Source: CAD feature listing. Evaluate the final solid. Frame: model axes, mm. A direction names the side the tool comes from. Round coordinates to 2 decimals unless told otherwise and drop trailing zeros. Loops run counter-clockwise (first coordinate to the right, second up) from the corner with the lowest first, then second, coordinate; pieces in that order, holes last. Notation, with made-up numbers: (34.25, 22) - (53.25, 22) arc R30 cw to (53.25, 45) - close; hole circle Ø8 at (12, 25). An arc over 180 degrees is marked (long way). Use CSV: the item, a comma, the result in double quotes. Start each with the question number.
from build123d import *

# Parameters (mm, degrees)
F1_DEPTH = 3.048
F3_DEPTH = 3.048
F5_DEPTH = 3.048


with BuildPart() as f1:
    # F0 (on Front) → F1 (new body)
    with BuildSketch(Plane.XZ):
        with BuildLine():
            Line((-27.215604, 61.783131), (-27.215604, -68.822387))
            ThreePointArc((-27.215604, -68.822387), (-26.099681, -71.516464), (-23.405604, -72.632387))
            Line((-23.405604, -72.632387), (-2.464669, -72.632387))
            Line((-2.464669, -72.632387), (-2.464669, -64.140432))
            Line((-2.464669, -64.140432), (-24.693408, -64.140432))
            ThreePointArc((-24.693408, -64.140432), (-25.232223, -63.917247), (-25.455408, -63.378432))
            Line((-25.455408, -63.378432), (-25.455408, -25.846069))
            ThreePointArc((-25.455408, -25.846069), (-25.232223, -25.307254), (-24.693408, -25.084069))
            Line((-24.693408, -25.084069), (-2.464669, -25.084069))
            Line((-2.464669, -25.084069), (-2.464669, -19.391987))
            Line((-2.464669, -19.391987), (-5.690682, -19.391987))
            ThreePointArc((-5.690682, -19.391987), (-6.229498, -19.168803), (-6.452682, -18.629987))
            Line((-6.452682, -18.629987), (-6.452682, 29.59835))
            ThreePointArc((-6.452682, 29.59835), (-6.229498, 30.137166), (-5.690682, 30.36035))
            Line((-5.690682, 30.36035), (-2.287077, 30.36035))
            Line((-2.287077, 30.36035), (-2.287077, 65.593131))
            Line((-2.287077, 65.593131), (-23.405604, 65.593131))
            ThreePointArc((-23.405604, 65.593131), (-26.099681, 64.477208), (-27.215604, 61.783131))
        make_face()
        with BuildLine():
            ThreePointArc((-25.455408, 8.798287), (-25.232223, 9.337102), (-24.693408, 9.560287))
            Line((-24.693408, 9.560287), (-17.513451, 9.560287))
            ThreePointArc((-17.513451, 9.560287), (-16.974636, 9.337102), (-16.751451, 8.798287))
            Line((-16.751451, 8.798287), (-16.751451, -1.699802))
            ThreePointArc((-16.751451, -1.699802), (-16.974636, -2.238618), (-17.513451, -2.461802))
            Line((-17.513451, -2.461802), (-24.693408, -2.461802))
            ThreePointArc((-24.693408, -2.461802), (-25.232223, -2.238618), (-25.455408, -1.699802))
            Line((-25.455408, -1.699802), (-25.455408, 8.798287))
        make_face(mode=Mode.SUBTRACT)
        with BuildLine():
            ThreePointArc((-25.455408, -7.460729), (-25.232223, -6.921914), (-24.693408, -6.698729))
            Line((-24.693408, -6.698729), (-16.028815, -6.698729))
            ThreePointArc((-16.028815, -6.698729), (-15.49, -6.475544), (-15.266815, -5.936729))
            Line((-15.266815, -5.936729), (-15.266815, 26.060438))
            ThreePointArc((-15.266815, 26.060438), (-15.043631, 26.599254), (-14.504815, 26.822438))
            Line((-14.504815, 26.822438), (-10.855766, 26.822438))
            ThreePointArc((-10.855766, 26.822438), (-10.316951, 26.599254), (-10.093766, 26.060438))
            Line((-10.093766, 26.060438), (-10.093766, -18.629987))
            ThreePointArc((-10.093766, -18.629987), (-10.316951, -19.168803), (-10.855766, -19.391987))
            Line((-10.855766, -19.391987), (-24.693408, -19.391987))
            ThreePointArc((-24.693408, -19.391987), (-25.232223, -19.168803), (-25.455408, -18.629987))
            Line((-25.455408, -18.629987), (-25.455408, -7.460729))
        make_face(mode=Mode.SUBTRACT)
        with BuildLine():
            ThreePointArc((-25.455408, 26.060438), (-25.232223, 26.599254), (-24.693408, 26.822438))
            Line((-24.693408, 26.822438), (-17.451537, 26.822438))
            ThreePointArc((-17.451537, 26.822438), (-16.912722, 26.599254), (-16.689537, 26.060438))
            Line((-16.689537, 26.060438), (-16.689537, 15.614866))
            ThreePointArc((-16.689537, 15.614866), (-16.912722, 15.07605), (-17.451537, 14.852866))
            Line((-17.451537, 14.852866), (-24.693408, 14.852866))
            ThreePointArc((-24.693408, 14.852866), (-25.232223, 15.07605), (-25.455408, 15.614866))
            Line((-25.455408, 15.614866), (-25.455408, 26.060438))
        make_face(mode=Mode.SUBTRACT)
        with BuildLine():
            Line((-25.455408, 31.034609), (-25.455408, 56.824335))
            ThreePointArc((-25.455408, 56.824335), (-25.232223, 57.36315), (-24.693408, 57.586335))
            Line((-24.693408, 57.586335), (-6.186478, 57.586335))
            ThreePointArc((-6.186478, 57.586335), (-5.647663, 57.36315), (-5.424478, 56.824335))
            Line((-5.424478, 56.824335), (-5.424478, 37.310197))
            ThreePointArc((-5.424478, 37.310197), (-5.647663, 36.771382), (-6.186478, 36.548197))
            Line((-6.186478, 36.548197), (-10.055168, 36.548197))
            ThreePointArc((-10.055168, 36.548197), (-10.593984, 36.325013), (-10.817168, 35.786197))
            Line((-10.817168, 35.786197), (-10.817168, 31.034609))
            ThreePointArc((-10.817168, 31.034609), (-11.040353, 30.495793), (-11.579168, 30.272609))
            Line((-11.579168, 30.272609), (-24.693408, 30.272609))
            ThreePointArc((-24.693408, 30.272609), (-25.232223, 30.495793), (-25.455408, 31.034609))
        make_face(mode=Mode.SUBTRACT)
        with BuildLine():
            Line((-1.799683, -19.391987), (-1.799683, -72.632387))
            Line((-1.799683, -72.632387), (22.221839, -72.632387))
            ThreePointArc((22.221839, -72.632387), (24.915916, -71.516464), (26.031839, -68.822387))
            Line((26.031839, -68.822387), (26.031839, 61.783131))
            ThreePointArc((26.031839, 61.783131), (24.915916, 64.477208), (22.221839, 65.593131))
            Line((22.221839, 65.593131), (-1.654555, 65.593131))
            Line((-1.654555, 65.593131), (-1.654555, 57.586335))
            Line((-1.654555, 57.586335), (22.565058, 57.586335))
            ThreePointArc((22.565058, 57.586335), (23.103874, 57.36315), (23.327058, 56.824335))
            Line((23.327058, 56.824335), (23.327058, 37.38084))
            ThreePointArc((23.327058, 37.38084), (23.103874, 36.842025), (22.565058, 36.61884))
            Line((22.565058, 36.61884), (-1.516778, 36.61884))
            Line((-1.516778, 36.61884), (-1.516778, 30.44359))
            Line((-1.516778, 30.44359), (4.297159, 30.44359))
            ThreePointArc((4.297159, 30.44359), (4.835975, 30.220406), (5.059159, 29.68159))
            Line((5.059159, 29.68159), (5.059159, -18.629987))
            ThreePointArc((5.059159, -18.629987), (4.835975, -19.168803), (4.297159, -19.391987))
            Line((4.297159, -19.391987), (-1.799683, -19.391987))
        make_face()
        with BuildLine():
            Line((23.327058, -19.723452), (23.327058, -63.378432))
            ThreePointArc((23.327058, -63.378432), (23.103874, -63.917247), (22.565058, -64.140432))
            Line((22.565058, -64.140432), (4.102913, -64.140432))
            ThreePointArc((4.102913, -64.140432), (3.564097, -63.917247), (3.340913, -63.378432))
            Line((3.340913, -63.378432), (3.340913, -26.143166))
            ThreePointArc((3.340913, -26.143166), (3.564097, -25.604351), (4.102913, -25.381166))
            Line((4.102913, -25.381166), (8.884725, -25.381166))
            Line((8.884725, -25.381166), (8.884725, -19.723452))
            ThreePointArc((8.884725, -19.723452), (9.10791, -19.184637), (9.646725, -18.961452))
            Line((9.646725, -18.961452), (22.565058, -18.961452))
            ThreePointArc((22.565058, -18.961452), (23.103874, -19.184637), (23.327058, -19.723452))
        make_face(mode=Mode.SUBTRACT)
        with BuildLine():
            Line((16.206523, -3.277048), (22.565058, -3.277048))
            ThreePointArc((22.565058, -3.277048), (23.103874, -3.500233), (23.327058, -4.039048))
            Line((23.327058, -4.039048), (23.327058, -14.328273))
            ThreePointArc((23.327058, -14.328273), (23.103874, -14.867088), (22.565058, -15.090273))
            Line((22.565058, -15.090273), (16.206523, -15.090273))
            ThreePointArc((16.206523, -15.090273), (15.667707, -14.867088), (15.444523, -14.328273))
            Line((15.444523, -14.328273), (15.444523, -4.039048))
            ThreePointArc((15.444523, -4.039048), (15.667707, -3.500233), (16.206523, -3.277048))
        make_face(mode=Mode.SUBTRACT)
        with BuildLine():
            Line((9.334675, 30.473812), (22.565058, 30.473812))
            ThreePointArc((22.565058, 30.473812), (23.103874, 30.250627), (23.327058, 29.711812))
            Line((23.327058, 29.711812), (23.327058, 18.880225))
            ThreePointArc((23.327058, 18.880225), (23.103874, 18.34141), (22.565058, 18.118225))
            Line((22.565058, 18.118225), (14.499665, 18.118225))
            ThreePointArc((14.499665, 18.118225), (13.96085, 17.89504), (13.737665, 17.356225))
            Line((13.737665, 17.356225), (13.737665, -14.725744))
            ThreePointArc((13.737665, -14.725744), (13.514481, -15.264559), (12.975665, -15.487744))
            Line((12.975665, -15.487744), (9.334675, -15.487744))
            ThreePointArc((9.334675, -15.487744), (8.79586, -15.264559), (8.572675, -14.725744))
            Line((8.572675, -14.725744), (8.572675, 29.711812))
            ThreePointArc((8.572675, 29.711812), (8.79586, 30.250627), (9.334675, 30.473812))
        make_face(mode=Mode.SUBTRACT)
        with BuildLine():
            Line((15.88612, 14.02483), (22.565058, 14.02483))
            ThreePointArc((22.565058, 14.02483), (23.103874, 13.801646), (23.327058, 13.26283))
            Line((23.327058, 13.26283), (23.327058, 2.677905))
            ThreePointArc((23.327058, 2.677905), (23.103874, 2.139089), (22.565058, 1.915905))
            Line((22.565058, 1.915905), (15.88612, 1.915905))
            ThreePointArc((15.88612, 1.915905), (15.347304, 2.139089), (15.12412, 2.677905))
            Line((15.12412, 2.677905), (15.12412, 13.26283))
            ThreePointArc((15.12412, 13.26283), (15.347304, 13.801646), (15.88612, 14.02483))
        make_face(mode=Mode.SUBTRACT)
    extrude(amount=F1_DEPTH)

    # F2 (on Front) → F3 (join)
    with BuildSketch(Plane.XZ):
        with BuildLine():
            Line((-25.056604, -74.105591), (23.872839, -74.105591))
            ThreePointArc((23.872839, -74.105591), (26.566916, -72.989667), (27.682839, -70.295591))
            Line((27.682839, -70.295591), (27.682839, 63.256334))
            ThreePointArc((27.682839, 63.256334), (26.566916, 65.950411), (23.872839, 67.066334))
            Line((23.872839, 67.066334), (-25.056604, 67.066334))
            ThreePointArc((-25.056604, 67.066334), (-27.750681, 65.950411), (-28.866604, 63.256334))
            Line((-28.866604, 63.256334), (-28.866604, -70.295591))
            ThreePointArc((-28.866604, -70.295591), (-27.750681, -72.989667), (-25.056604, -74.105591))
        make_face()
        with BuildLine():
            Line((-16.71073, -64.140432), (-24.693408, -64.140432))
            ThreePointArc((-24.693408, -64.140432), (-25.232223, -63.917247), (-25.455408, -63.378432))
            Line((-25.455408, -63.378432), (-25.455408, -25.846069))
            ThreePointArc((-25.455408, -25.846069), (-25.232223, -25.307254), (-24.693408, -25.084069))
            Line((-24.693408, -25.084069), (-16.71073, -25.084069))
            Line((-16.71073, -25.084069), (-16.71073, -64.140432))
        make_face(mode=Mode.SUBTRACT)
        with BuildLine():
            Line((-16.71073, 57.586335), (-16.71073, 30.272609))
            Line((-16.71073, 30.272609), (-24.693408, 30.272609))
            ThreePointArc((-24.693408, 30.272609), (-25.232223, 30.495793), (-25.455408, 31.034609))
            Line((-25.455408, 31.034609), (-25.455408, 56.824335))
            ThreePointArc((-25.455408, 56.824335), (-25.232223, 57.36315), (-24.693408, 57.586335))
            Line((-24.693408, 57.586335), (-16.71073, 57.586335))
        make_face(mode=Mode.SUBTRACT)
    extrude(amount=-F3_DEPTH)

    # F4 (on face) → F5 (join)
    with BuildSketch(Plane(origin=(0, 3.048, 0), x_dir=(-1, 0, 0), z_dir=(0, 1, 0))):
        with BuildLine():
            Line((-29.664039, 64.526334), (-29.664039, -71.565591))
            ThreePointArc((-29.664039, -71.565591), (-28.176141, -75.157693), (-24.584039, -76.645591))
            Line((-24.584039, -76.645591), (25.767804, -76.645591))
            ThreePointArc((25.767804, -76.645591), (29.359906, -75.157693), (30.847804, -71.565591))
            Line((30.847804, -71.565591), (30.847804, 64.526334))
            ThreePointArc((30.847804, 64.526334), (29.359906, 68.118437), (25.767804, 69.606334))
            Line((25.767804, 69.606334), (-24.584039, 69.606334))
            ThreePointArc((-24.584039, 69.606334), (-28.176141, 68.118437), (-29.664039, 64.526334))
        make_face()
    extrude(amount=F5_DEPTH)


solid = f1.part
1. Section query A-A on z = -27.5. Return the cut outline in (x, y).
2. Mould query, pull axis Z, two halves, no side actions, for faces 4 (the cylindrical face through (24.945, -1.503, 64.447)), 5 (the flat face through (-1.8, -2, -46)), 6 (the flat face through (-21, 0, 21)). Classes: +Z half, -Z half, draft (parallel to the pull), parting line (faces both ways), or undercut.
3. Reachability of faces 1 (the flat face through (-2.465, -2, -68)), 2 (the flat face through (-27.216, -2, -3)), 3 (the flat face through (-21, -2, -2.462)) from +Z, -Z, +X, -X, +Y, -Y: full face, straight path, thin tool, end or side. Return the list, or none.
4. Section query C-C on z = 43.5. Return the cut outline in (x, y).
5. Line query: line 1 along Z through (x, y) = (-22.5, 1.5); line 2 along Z through (x, y) = (-7.5, -2); line 3 along X through (y, z) = (-1.75, -10). Output: solid intervals per line, ascending.
6. Section query D-D on x = 7. Return the cut outline in (y, z).
7. Contact query for flat-ended pins moving along their axis: P1, Ø2.5, axis at x = 2, y = -1, coming from the -Z side; P2, Ø1.5, axis at y = -1.5, z = -36.5, coming from the +X side; P3, Ø1.5, axis at y = -0.5, z = 37.5, coming from the +X side. Output: stop coordinate, or through.
Values:
1,outline,"(-30.85, 3.05) - (-28.87, 3.05) - (-28.87, 0) - (-27.22, 0) - (-27.22, -3.05) - (-25.46, -3.05) - (-25.46, 3.05) - (-16.71, 3.05) - (-16.71, 0) - (-1.8, 0) - (-1.8, -3.05) - (3.34, -3.05) - (3.34, 0) - (23.33, 0) - (23.33, -3.05) - (26.03, -3.05) - (26.03, 0) - (27.68, 0) - (27.68, 3.05) - (29.66, 3.05) - (29.66, 6.1) - (-30.85, 6.1) - close"
2,face 4,"+Z half"
2,face 5,"draft"
2,face 6,"undercut"
3,face 1,"-Z, -Y"
3,face 2,"+Z, -Z, -X, -Y"
3,face 3,"-Y"
4,outline,"(-30.85, 3.05) - (-28.87, 3.05) - (-28.87, 0) - (-27.22, 0) - (-27.22, -3.05) - (-25.46, -3.05) - (-25.46, 3.05) - (-16.71, 3.05) - (-16.71, 0) - (-5.42, 0) - (-5.42, -3.05) - (-2.29, -3.05) - (-2.29, 0) - (23.33, 0) - (23.33, -3.05) - (26.03, -3.05) - (26.03, 0) - (27.68, 0) - (27.68, 3.05) - (29.66, 3.05) - (29.66, 6.1) - (-30.85, 6.1) - close"
5,line 1,"z = -74.11 to -64.14, -25.08 to 30.27, 57.59 to 67.07"
5,line 2,"z = -72.63 to -64.14, -25.08 to 36.55, 57.59 to 65.59"
5,line 3,"x = -27.22 to -25.46, -10.09 to -6.45, 5.06 to 8.57, 13.74 to 15.44, 23.33 to 26.03"
6,outline,"(-3.05, -72.63) - (0, -72.63) - (0, -74.11) - (3.05, -74.11) - (3.05, -76.65) - (6.1, -76.65) - (6.1, 69.61) - (3.05, 69.61) - (3.05, 67.07) - (0, 67.07) - (0, 65.59) - (-3.05, 65.59) - (-3.05, 57.59) - (0, 57.59) - (0, 36.62) - (-3.05, 36.62) - (-3.05, -25.38) - (0, -25.38) - (0, -64.14) - (-3.05, -64.14) - close"
7,P1,"stops at z = -74.11"
7,P2,"stops at x = 26.03"
7,P3,"stops at x = 27.68"
